```python
from build123d import *

# Parameters (mm, degrees)
EXTRUDE_1_DEPTH     = 30
SKETCH_2_R          = 34
CUT_EXTRUDE_1_DEPTH = 116.758369028
CUT_EXTRUDE_2_DEPTH = 20


with BuildPart() as part:
    # 草圖1 → 填料-伸長1 (new body)
    with BuildSketch(Plane.XY):
        Polygon((-50, -30), (50, -30), (50, 30), (37.5, 30), (37.5, 100), (-37.5, 100), (-37.5, 30), (-50, 30), align=None)
    extrude(amount=EXTRUDE_1_DEPTH)

    # 草圖2 → 除料-伸長1 (cut, through all)
    with BuildSketch(Plane.XY.offset(30)):
        with Locations((0, 50)):
            Circle(SKETCH_2_R)
    extrude(amount=-CUT_EXTRUDE_1_DEPTH, mode=Mode.SUBTRACT)

    # 草圖3 → 除料-伸長2 (cut)
    with BuildSketch(Plane.XY.offset(30)):
        with BuildLine():
            Line((-45, -25), (-7, -25))
            Line((-7, -25), (-7, 16.728390481))
            ThreePointArc((-7, 16.728390481), (-22.925968466, 24.892232877), (-32.5, 40.012507822))
            Line((-32.5, 40.012507822), (-32.5, 25))
            Line((-32.5, 25), (-45, 25))
            Line((-45, 25), (-45, -25))
        make_face()
    cut_extrude_2 = extrude(amount=-CUT_EXTRUDE_2_DEPTH, mode=Mode.SUBTRACT)

    # 鏡射1: 除料-伸長2 across plane
    add(cut_extrude_2.mirror(Plane(origin=(0, 0, 0), x_dir=(0, 0, 1), z_dir=(1, 0, 0))), mode=Mode.SUBTRACT)


solid = part.part
```
The listing builds one solid part. Answer for the finished solid, in the listing's coordinates (mm). A direction names the side the tool comes from. Round coordinates to 2 decimals unless told otherwise and drop trailing zeros. Loops run counter-clockwise (first coordinate to the right, second up) from the corner with the lowest first, then second, coordinate; pieces in that order, holes last. Notation, with made-up numbers: (19.5, 74) -> (59.5, 74) arc R21 ccw to (59.5, 85) -> close; hole circle Ø2 at (81, 35.5). An arc over 180 degrees is marked (long way). Use one line per item in the form item = value.
1. The part is cut by section A-A on x = 0. Determine the outline of the cut face in (y, z).
Answer key:
outline = (-30, 0) -> (16, 0) -> (16, 30) -> (-30, 30) -> close; (84, 0) -> (100, 0) -> (100, 30) -> (84, 30) -> close
2. The part is cut by section C-C on z = 22. Determine the outline of the cut face in (x, y), and give its area (3 significant figures).
Answer key:
outline = (-50, -30) -> (50, -30) -> (50, 30) -> (37.5, 30) -> (37.5, 100) -> (-37.5, 100) -> (-37.5, 30) -> (-50, 30) -> close; hole (-45, -25) -> (-7, -25) -> (-7, 16.73) arc R34 ccw to (7, 16.73) -> (7, -25) -> (45, -25) -> (45, 25) -> (32.5, 25) -> (32.5, 40.01) arc R34 ccw (long way) to (-32.5, 40.01) -> (-32.5, 25) -> (-45, 25) -> close
area = 3,870 mm²
3. Find the intervals of material crossed by probe 1 along X at (y, z) = (-19, 27.75); probe 2 along X at (y, z) = (50, 17); probe 3 along Y at (x, z) = (37, 22.5), in increasing order. Write a range as [from, to].
Answer key:
probe_1 = [-50, -45], [-7, 7], [45, 50]
probe_2 = [-37.5, -34], [34, 37.5]
probe_3 = [-30, -25], [25, 100]
4. Flat-ended cylindrical pins translate along their axes: pin 1 Ø5 at (y, z) = (83, 26.5) entering from -X; pin 2 Ø11.5 at (x, y) = (-24.5, 17.5) entering from +Z; pin 3 Ø12 at (y, z) = (42.5, 23.5) entering from +X. Find the tip coordinate at first contact, or state that the pin passes through.
Answer key:
pin_1 = -37.5
pin_2 = 10
pin_3 = 37.5
5. The part is cut by section D-D on x = 41.5. Determine the outline of the cut face in (y, z).
Answer key:
outline = (-30, 0) -> (30, 0) -> (30, 30) -> (25, 30) -> (25, 10) -> (-25, 10) -> (-25, 30) -> (-30, 30) -> close
6. A tool of negligible diameter and unlimited length cuts with its end or side. For faces 1 (the flat face through (44, 30, 15)), 2 (the flat face through (-44, 30, 15)), 3 (the flat face through (32.5, 33, 20)), from which of +Z, -Z, +X, -X, +Y, -Y can it reach the whole face along a straight path? Write none if from no direction.
Answer key:
face_1 = +Z, -Z, +X, +Y
face_2 = +Z, -Z, -X, +Y
face_3 = +Z
7. The part is cut by section B-B on y = 50. Determine the outline of the cut face in (x, z), and give its area (3 significant figures).
Answer key:
outline = (-37.5, 0) -> (-34, 0) -> (-34, 30) -> (-37.5, 30) -> close; (34, 0) -> (37.5, 0) -> (37.5, 30) -> (34, 30) -> close
area = 210 mm²
8. For a pull along X with two mould halves and no side action, classify faces 4 (the flat face through (-37.5, 65, 15)), 5 (the flat face through (-26, 1, 10)), 6 (the flat face through (37.5, 65, 15)), 7 (the flat face through (-4, 16, 30)) as released by +X, released by -X, zero draft, split by the parting line, or undercut.
Answer key:
face_4 = released by -X
face_5 = undercut
face_6 = released by +X
face_7 = zero draft
